Geometry: final body of the model. Coordinates: model frame, mm. Give positions to 0.01 mm unless a question says otherwise; leave off trailing zeros. Order: outer loops, then holes, each group sorted by start corner. A loop starts at its lowest first (then second) coordinate and runs counter-clockwise, first axis right, second up. Notation, with made-up numbers: (57, 84) -> (114, 84) arc R12 ccw to (114, 96) -> close; hole circle Ø3 at (65, 56). An arc over 180 degrees is marked (long way). Write item = value, one per line.
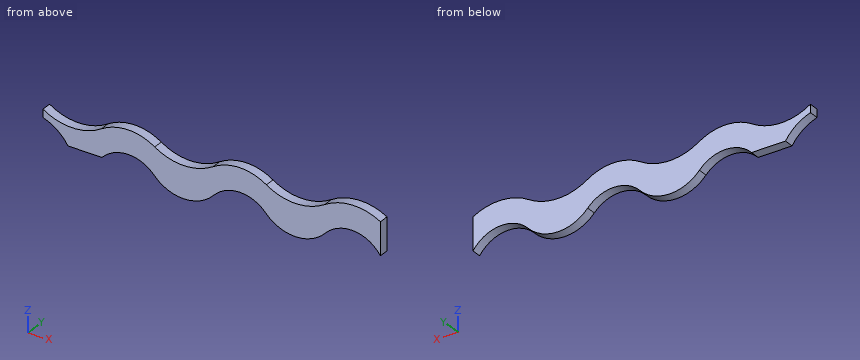
```python
from build123d import *

# Parameters (mm, degrees)
BOSS_EXTRUDE1_DEPTH = 2


with BuildPart() as part:
    # Sketch2 → Boss-Extrude1 (new body)
    with BuildSketch(Plane(origin=(0, 0, 0), x_dir=(1, 0, 0), z_dir=(0, 1, 0))):
        with BuildLine():
            Line((63.346978543, 15.774727996), (63.346978543, 9.034727996))
            ThreePointArc((63.346978543, 9.034727996), (57.571540875, 7.622708087), (51.89, 9.374727996))
            ThreePointArc((51.89, 9.374727996), (45.9, 11.125), (39.91, 9.374727996))
            ThreePointArc((39.91, 9.374727996), (34.425, 7.772016487), (28.94, 9.374727996))
            ThreePointArc((28.94, 9.374727996), (22.95, 11.125), (16.96, 9.374727996))
            ThreePointArc((16.96, 9.374727996), (11.475, 7.772016487), (5.99, 9.374727996))
            ThreePointArc((5.99, 9.374727996), (0, 11.125), (-5.99, 9.374727996))
            Line((-5.99, 9.374727996), (-5.99, 11.044727996))
            ThreePointArc((-5.99, 11.044727996), (-3.073533572, 12.552842644), (-0.867605229, 14.984727996))
            Line((-0.867605229, 14.984727996), (6.120538735, 14.984727996))
            ThreePointArc((6.120538735, 14.984727996), (11.47, 12.62816893), (16.819461265, 14.984727996))
            ThreePointArc((16.819461265, 14.984727996), (22.945, 17.683166797), (29.070538735, 14.984727996))
            ThreePointArc((29.070538735, 14.984727996), (34.42, 12.62816893), (39.769461265, 14.984727996))
            ThreePointArc((39.769461265, 14.984727996), (45.895, 17.683166797), (52.020538735, 14.984727996))
            ThreePointArc((52.020538735, 14.984727996), (57.874449684, 12.645739842), (63.346978543, 15.774727996))
        make_face()
    extrude(amount=BOSS_EXTRUDE1_DEPTH)


solid = part.part
```
1) Line query: line 1 (X direction, y = 1.8, z = -13.75); line 2 (X direction, y = 0.9, z = -14); line 3 (X direction, y = 1.8, z = -15.25). Output: solid intervals per line, ascending. Write a range as from..to.
Check sheet entries:
line_1 = -1.79..7.6, 15.34..30.55, 38.29..53.5, 61.24..63.35
line_2 = -1.58..7.23, 15.71..30.18, 38.66..53.13, 61.61..63.35
line_3 = 17.07..28.82, 40.02..51.77, 62.95..63.35
2) Section query B-B (y = 0.3). Output: boundary loops of the cut face in (x, z) (3 decimals).
Check sheet entries:
outline = (-5.99, -11.045) arc R9.25 cw to (-0.868, -14.985) -> (6.121, -14.985) arc R7.25 cw to (16.819, -14.985) arc R8.302 ccw to (29.071, -14.985) arc R7.25 cw to (39.769, -14.985) arc R8.302 ccw to (52.021, -14.985) arc R7.25 cw to (63.347, -15.775) -> (63.347, -9.035) arc R11.167 ccw to (51.89, -9.375) arc R11.125 cw to (39.91, -9.375) arc R10.187 ccw to (28.94, -9.375) arc R11.125 cw to (16.96, -9.375) arc R10.187 ccw to (5.99, -9.375) arc R11.125 cw to (-5.99, -9.375) -> close
3) Section query D-D (x = 26.5). Output: boundary loops of the cut face in (y, z), plus the area to 3 significant figures.
Check sheet entries:
outline = (0, -16.88) -> (2, -16.88) -> (2, -10.54) -> (0, -10.54) -> close
area = 12.7 mm²
4) Section query A-A (z = -14). Output: boundary loops of the cut face in (x, y), plus the area to 3 significant figures.
Check sheet entries:
outline = (-1.58, 0) -> (7.23, 0) -> (7.23, 2) -> (-1.58, 2) -> close; (15.71, 0) -> (30.18, 0) -> (30.18, 2) -> (15.71, 2) -> close; (38.66, 0) -> (53.13, 0) -> (53.13, 2) -> (38.66, 2) -> close; (61.61, 0) -> (63.35, 0) -> (63.35, 2) -> (61.61, 2) -> close
area = 78.9 mm²
5) First-contact query: P1, Ø1, axis at y = 0, z = -16, coming from the -X side; P2, Ø1, axis at x = 2, y = 1.5, coming from the -Z side. Flat tips, straight axial feed; report the tip coordinate or a pass-through.
Check sheet entries:
P1 = 17.33
P2 = -14.98
6) Section query C-C (x = 55.5). Output: boundary loops of the cut face in (y, z), plus the area to 3 significant figures.
Check sheet entries:
outline = (0, -12.87) -> (2, -12.87) -> (2, -7.88) -> (0, -7.88) -> close
area = 9.99 mm²
